from build123d import *

# Parameters (mm, degrees)
SKETCH_1_R          = 5
SKETCH_1_R_2        = 2.7
EXTRUDE_1_DEPTH     = 14
EXTRUDE_START       = -14
EXTRUDE_2_DEPTH     = 14
SKETCH_5_W          = 6.3
SKETCH_5_H          = 2.5
CUT_EXTRUDE_3_DEPTH = 10
SKETCH_10_W         = 11.05826702
SKETCH_10_H         = 10.05
CUT_EXTRUDE_5_DEPTH = 9.4
SKETCH_12_R         = 1.6
CUT_EXTRUDE_7_DEPTH = 23.639691363


with BuildPart() as part:
    # Эскиз1 → Бобышка-Вытянуть1 (new body)
    with BuildSketch(Plane.XY):
        Circle(SKETCH_1_R)
        Circle(SKETCH_1_R_2, mode=Mode.SUBTRACT)
    extrude(amount=EXTRUDE_1_DEPTH)

    # Эскиз2 → Бобышка-Вытянуть2 (add)
    with BuildSketch(Plane.XY.offset(14).offset(EXTRUDE_START)):
        with BuildLine():
            Line((-5, 0), (-2.7, 0))
            ThreePointArc((-2.7, 0), (0, 2.7), (2.7, 0))
            Line((2.7, 0), (5, 0))
            Line((5, 0), (5, 20))
            Line((5, 20), (-5, 20))
            Line((-5, 20), (-5, 0))
        make_face()
    extrude(amount=EXTRUDE_2_DEPTH)

    # Эскиз5 → Вырез-Вытянуть3 (cut)
    with BuildSketch(Plane.XY.offset(14)):
        with Locations((0.1, 16.5)):
            Rectangle(SKETCH_5_W, SKETCH_5_H)
    extrude(amount=-CUT_EXTRUDE_3_DEPTH, mode=Mode.SUBTRACT)

    # Эскиз10 → Вырез-Вытянуть5 (cut)
    with BuildSketch(Plane.ZY.offset(5)):
        with Locations((6.97086649, 7.95)):
            Rectangle(SKETCH_10_W, SKETCH_10_H)
    extrude(amount=-CUT_EXTRUDE_5_DEPTH, mode=Mode.SUBTRACT)

    # Эскиз12 → Вырез-Вытянуть7 (cut, through all)
    with BuildSketch(Plane(origin=(0, 2.925, 0), x_dir=(1, 0, 0), z_dir=(0, 1, 0))):
        with Locations(Location((0.19946897, -6.97086649, 0), (0, 0, 90))):
            Circle(SKETCH_12_R)
    extrude(amount=CUT_EXTRUDE_7_DEPTH, mode=Mode.SUBTRACT)


solid = part.part
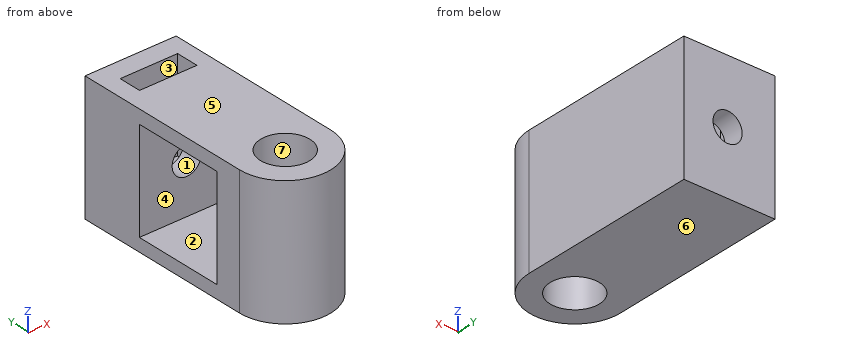
Read the model definition and answer for the solid it produces. Units are mm, in the model's axes. Face numbers are marked on the shaded views. A direction names the side the tool comes from. Round coordinates to 2 decimals unless told otherwise and drop trailing zeros. Loops run counter-clockwise (first coordinate to the right, second up) from the corner with the lowest first, then second, coordinate; pieces in that order, holes last.
Q1. Determine the mould class of the marked faces 4, 5, 6 and 7 for opening direction Z: released by +Z, released by -Z, zero draft, split by the parting line, or undercut.
Q2. Section B-B on y = 6 is taken. Write down the section's boundary in (x, z).
Q3. This flat-tipped pin is pushed along its axis until it touches: pin 1 (5 mm diameter, centred on y = 7, z = 5, fed in from -X). Where does it stop, or does it pass through?
Q4. Section C-C on x = 0.5 is taken. Write down the section's boundary in (y, z) (3 decimals).
Q5. Section D-D on z = 11 is taken. Write down the section's boundary in (x, y) (3 decimals), and give its area (3 significant figures).
Q6. Section A-A on z = 7.5 is taken. Give the number of separate pieces and of enclosed holes in the cut face, and give its area (3 significant figures).
Q7. Which of the six approach directions +Z, -Z, +X, -X, +Y, -Y give full straight-line access (tool end or side, diameter ignored) to the marked faces 1, 2 and 3?
Q8. Consider probe 1 along X at (y, z) = (17, 6.75); probe 2 along Z at (x, y) = (-1.25, 7.75); probe 3 along Y at (x, z) = (-0.25, 3) (3 decimals). Determine where each line is inside the solid, lowest interval first.
Output:
1. face 4: undercut
1. face 5: released by +Z
1. face 6: released by -Z
1. face 7: zero draft
2. outline: (-5, 0) - (5, 0) - (5, 14) - (-5, 14) - (-5, 12.5) - (4.4, 12.5) - (4.4, 1.44) - (-5, 1.44) - close
3. pin 1: stops at x = 4.4
4. outline: (-4.975, 0) - (-2.653, 0) - (-2.653, 14) - (-4.975, 14) - close; (2.653, 0) - (20, 0) - (20, 5.399) - (17.75, 5.399) - (17.75, 4) - (15.25, 4) - (15.25, 5.399) - (12.975, 5.399) - (12.975, 1.442) - (2.925, 1.442) - (2.925, 12.5) - (12.975, 12.5) - (12.975, 8.542) - (15.25, 8.542) - (15.25, 14) - (2.653, 14) - close; (17.75, 8.542) - (20, 8.542) - (20, 14) - (17.75, 14) - close
5. outline: (-5, 0) arc R5 ccw to (5, 0) - (5, 20) - (-5, 20) - (-5, 12.975) - (4.4, 12.975) - (4.4, 2.925) - (-5, 2.925) - close; hole (-3.05, 15.25) - (3.25, 15.25) - (3.25, 17.75) - (-3.05, 17.75) - close; hole circle Ø5.4 at (0, 0)
5. area: 106 mm2
6. separate pieces: 2
6. enclosed holes: 1
6. area: 92.5 mm2
7. face 1: +Y
7. face 2: -X
7. face 3: +Z
8. probe 1: x = -5 to -3.05, 3.25 to 5
8. probe 2: z = 0 to 1.44, 12.5 to 14
8. probe 3: y = -4.994 to -2.688, 2.688 to 2.925, 12.975 to 20
